```python
from build123d import *

# Parameters (mm, degrees)
F1_DEPTH = 483.87
F2_R     = 63.5
F3_DEPTH = 307.34
F4_R     = 38.1
F5_DEPTH = 170.18


with BuildPart() as f1:
    # F0 (on Front) → F1 (new body)
    with BuildSketch(Plane.XZ):
        with BuildLine():
            Line((-5.7769804876, 250.2069493125), (-39.9019537476, 284.3319225726))
            Line((-39.9019537476, 284.3319225726), (-488.9147598011, -164.6808834809))
            ThreePointArc((-488.9147598011, -164.6808834809), (-513.1412824891, -286.4758377474), (-409.8885059357, -355.4671373463))
            Line((-409.8885059357, -355.4671373463), (860.1114940643, -355.4671373463))
            Line((860.1114940643, -355.4671373463), (860.1114940643, -307.2071373463))
            Line((860.1114940643, -307.2071373463), (-409.8885059357, -307.2071373463))
            ThreePointArc((-409.8885059357, -307.2071373463), (-447.9966898633, -238.4179483219), (-420.664813281, -164.6808834809))
            Line((-420.664813281, -164.6808834809), (-5.7769804876, 250.2069493125))
        make_face()
    extrude(amount=F1_DEPTH)

    # F2 (on face) → F3 (cut)
    with BuildSketch(Plane.XY.offset(-307.2071373463)):
        with Locations((47.3114940643, -241.5729016066)):
            Circle(F2_R)
        with BuildLine():
            Line((758.6122675238, -174.8664157407), (504.6122675238, -174.8664157407))
            ThreePointArc((504.6122675238, -174.8664157407), (441.1122675238, -238.3664157407), (504.6122675238, -301.8664157407))
            Line((504.6122675238, -301.8664157407), (758.6122675238, -301.8664157407))
            ThreePointArc((758.6122675238, -301.8664157407), (822.1122675238, -238.3664157407), (758.6122675238, -174.8664157407))
        make_face()
    extrude(amount=-F3_DEPTH, mode=Mode.SUBTRACT)

    # F4 (on face) → F5 (cut)
    with BuildSketch(Plane(origin=(-162.1169381601, 0, 162.1169381601), x_dir=(0, -1, 0), z_dir=(-0.7071067812, 0, 0.7071067812))):
        with Locations((114.3, -17.6619115186)):
            Circle(F4_R)
        with Locations((369.57, -17.6619115186)):
            Circle(F4_R)
    extrude(amount=-F5_DEPTH, mode=Mode.SUBTRACT)


solid = f1.part
```
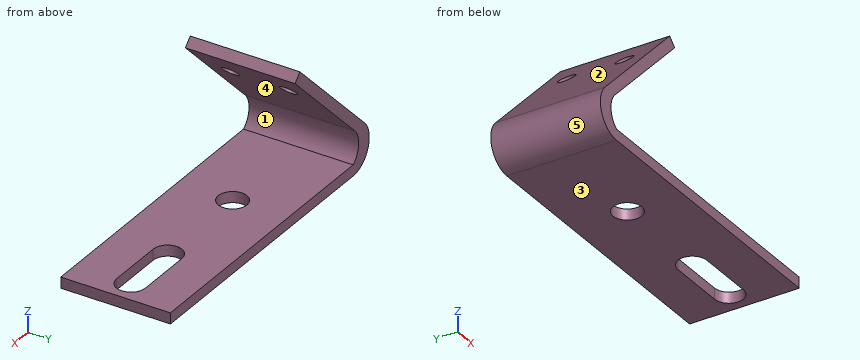
The listing builds one solid part. Answer for the finished solid, in the listing's coordinates (mm). Face numbers are marked on the shaded views. A direction names the side the tool comes from. Coordinates: 2 decimals unless noted, no trailing zeros. Loops run counter-clockwise (first coordinate to the right, second up) from the corner with the lowest first, then second, coordinate; pieces in that order, holes last. Notation, with made-up numbers: M 56,0.25 L 93,0.25 A23 cw 93,35.25 Z; hole C 18.5,67.5 d9. An arc over 180 degrees is marked long. Answer as CSV lines item,"result". Start each with the question number.
(1) The part is cut by section D-D (z = -185.5). Give the vertices of the cut face in (x, y).
(2) Given pin 1 (3 mm diameter, centred on x = 83, y = -427, fed in from +Z); pin 2 (5 mm diameter, centred on x = -344.5, y = -293.5, fed in from +Z); pin 3 (10 mm diameter, centred on x = -97.5, y = -341, fed in from +Z), each flat-ended and moving along its own axis, determine where each tip first touches the part or whether it passes through.
(3) Find the intervals of material crossed by L1, parallel to Z at x = -269.5, y = -356; L2, parallel to Z at x = 37, y = -136.5; L3, parallel to X at y = -410.5, z = -132.5, in increasing order. Write a range as [from, to].
(4) For the marked faces 4 and 5, determine the directions among +Z, -Z, +X, -X, +Y, -Y from which every point of the face is accessible in a straight line to the end or side of a thin tool.
(5) The part is cut by section A-A (x = 536.5). Give the vertices of the cut face in (y, z), and give its area (3 significant figures).
(6) The part is cut by section C-C (x = 378). Give the vertices of the cut face in (y, z), and give its area (3 significant figures).
(7) The part is cut by section B-B (y = -371). Give the vertices of the cut face in (x, z), and give its area (3 significant figures).
(8) The mould has two halves that part along Z. Classify the marked faces 1, 2 and 3: pulls with the +Z half, pulls with the -Z half, needs draft (parallel to the pull), parting line crosses it, or undercut.
Determined:
1,outline,"M -505.29,-483.87 L -436.38,-483.87 L -436.38,0 L -505.29,0 Z"
2,pin 1,"z = -307.21"
2,pin 2,"z = -17.77"
2,pin 3,"z = 231.73"
3,L1,"[-355.47, -307.21], [-13.52, 54.73]"
3,L2,"[-355.47, -307.21]"
3,L3,"[-456.73, -388.48]"
4,face 4,"+X, +Y, -Y"
4,face 5,"-X, +Y, -Y"
5,outline,"M -483.87,-355.47 L -301.87,-355.47 L -301.87,-307.21 L -483.87,-307.21 Z; M -174.87,-355.47 L 0,-355.47 L 0,-307.21 L -174.87,-307.21 Z"
5,area,"17,200 mm2"
6,outline,"M -483.87,-355.47 L 0,-355.47 L 0,-307.21 L -483.87,-307.21 Z"
6,area,"23,400 mm2"
7,outline,"M -488.91,-164.68 A111.76 ccw -409.89,-355.47 L 860.11,-355.47 L 860.11,-307.21 L -409.89,-307.21 A94.23 cw -420.66,-164.68 L -167.4,88.58 L -201.53,122.71 Z; M -147.68,176.55 L -113.56,142.42 L -5.78,250.21 L -39.9,284.33 Z"
7,area,"101,000 mm2"
8,face 1,"undercut"
8,face 2,"pulls with the +Z half"
8,face 3,"pulls with the -Z half"
